Autodesk Inventor part; units mm, degrees
ref_plane "YZ Plane" through (0, 0, 0) normal (1, 0, 0) x (0, 1, 0)
ref_plane "XZ Plane" through (0, 0, 0) normal (0, 1, 0) x (-1, 0, 0)
ref_plane "XY Plane" through (0, 0, 0) normal (0, 0, 1) x (1, 0, 0)
sketch "Sketch3" plane through (0, 0, 0) normal (0, 1, 0) x (-1, 0, 0)
  line L0 (0.305195, 0) -> (-44.144805, 0)
  line L1 (-44.144805, 0) -> (-44.144805, -19.05)
  line L2 (-44.144805, -19.05) -> (0.305195, -19.05)
  line L3 (0.305195, -19.05) -> (0.305195, 0)
  arc A0 (-5.25, -6.73951) -> (-5.25, -5.26049) centre (-3.125, -6) ccw
  circle A1 centre (-3.125, -6) radius 2.25
  arc A2 (35.25, -5.26049) -> (35.25, -6.73951) centre (33.125, -6) ccw
  circle A3 centre (33.125, -6) radius 2.25
  line L4 (33.125, -6) -> (-3.125, -6)
  line L5 (0, -12) -> (0, 0)
  line L6 (30, -12) -> (0, -12)
  line L7 (0, -12) -> (0, 0)
  line L8 (0, 0) -> (30, 0)
  line L9 (30, 0) -> (30, -12)
  line L10 (30, -12) -> (0, 0) construction
  line L11 (0, -12) -> (30, 0) construction
  arc A4 (-42.475, -10.26451) -> (-42.475, -8.78549) centre (-40.35, -9.525) ccw
  circle A5 centre (-40.35, -9.525) radius 2.25
  arc A6 (-1.975, -8.78549) -> (-1.975, -10.26451) centre (-4.1, -9.525) ccw
  circle A7 centre (-4.1, -9.525) radius 2.25
  line L12 (-4.1, -9.525) -> (-40.35, -9.525)
  line L13 (-37.225, -15.525) -> (-37.225, -3.525)
  line L14 (-7.225, -15.525) -> (-37.225, -15.525)
  line L15 (-37.225, -15.525) -> (-37.225, -3.525)
  line L16 (-37.225, -3.525) -> (-7.225, -3.525)
  line L17 (-7.225, -3.525) -> (-7.225, -15.525)
  line L18 (-7.225, -15.525) -> (-37.225, -3.525) construction
  line L19 (-37.225, -15.525) -> (-7.225, -3.525) construction
  point P0 (15, -6)
  point P1 (-22.225, -9.525)
  point P2 (-4.875952, -7.413035)
  point P3 (-5.25, -6.73951)
  point P4 (-2.349048, -8.111965)
  point P5 (-1.975, -10.26451)
  point P6 (0.305195, -12)
  dimension "d12" = 4.5
  dimension "d13" = 4.5
  dimension "d17" = 4.5
  dimension "d18" = 4.5
  dimension "d9" = 44.45
  dimension "d10" = 19.05
  dimension "d11" = 36.25
  dimension "d14" = 30
  dimension "d15" = 12
  dimension "d16" = 36.25
  dimension "d19" = 30
  dimension "d20" = 12
extrude "Extrusion2" add sketch "Sketch3" along normal blind 3.81 contours L5 L6 L3 L2 L1 L0 | A0 A6 A1
sketch "Sketch4" plane through (0, 3.81, 0) normal (0, 1, 0) x (1, 0, 0)
  line L0 (0, 12) -> (0, 0)
  line L1 (-0.305195, 19.05) -> (-0.305195, 12)
  line L2 (0, 12) -> (-0.305195, 12)
  line L3 (-0.305195, 12) -> (-0.305195, 19.05)
  line L4 (-0.305195, 19.05) -> (0, 19.05)
  line L5 (0, 19.05) -> (0, 12)
extrude "Extrusion3" cut sketch "Sketch4" against normal blind 3.81
sketch "Sketch5" plane through (0, 3.81, 0) normal (0, 1, 0) x (1, 0, 0)
  line L0 (44.144805, 19.05) -> (0, 19.05)
  line L1 (22.072403, 19.05) -> (22.072403, 0)
  line L2 (0, 0) -> (44.144805, 0)
  line L3 (22.072403, 9.525) -> (0, 9.525)
  line L4 (0, 19.05) -> (0, 0)
  circle A0 centre (3.999998, -4) radius 4
  circle A1 centre (3.999998, -4) radius 1.5
  line L5 (0, 0) -> (44.144805, 0)
  line L6 (0, -4.004242) -> (0, 0)
  line L7 (0, 0) -> (7.846401, 0)
  line L8 (7.846401, 0) -> (7.999998, -4.001295)
  circle A2 centre (3.999998, 23.05) radius 4
  circle A3 centre (3.999998, 23.05) radius 1.5
  line L9 (0, 23.054242) -> (0, 19.05)
  line L10 (0, 19.05) -> (7.846401, 19.05)
  line L11 (7.846401, 19.05) -> (7.999998, 23.051295)
  line L12 (44.144805, 19.05) -> (44.144805, 0)
  circle A4 centre (40.144808, -4) radius 4
  circle A5 centre (40.144808, -4) radius 1.5
  line L13 (44.144805, -4.004242) -> (44.144805, 0)
  line L14 (44.144805, 0) -> (36.298405, 0)
  line L15 (36.298405, 0) -> (36.144808, -4.001295)
  circle A6 centre (40.144808, 23.05) radius 4
  circle A7 centre (40.144808, 23.05) radius 1.5
  line L16 (44.144805, 23.054242) -> (44.144805, 19.05)
  line L17 (44.144805, 19.05) -> (36.298405, 19.05)
  line L18 (36.298405, 19.05) -> (36.144808, 23.051295)
  point P0 (44.144805, 9.525)
  point P1 (7.846401, 0)
  dimension "d25" = 8
  dimension "d26" = 3
sketch "Sketch5 outline for Extrusion4" plane through (0, 3.81, 0) normal (0, 1, 0) x (1, 0, 0)
  line L0 (44.144805, -4.004242) -> (44.144805, 0)
  arc A0 (36.144808, -4.001295) -> (44.144805, -4.004242) centre (40.144808, -4) ccw
  line L1 (44.144805, 0) -> (36.298405, 0)
  line L2 (36.298405, 0) -> (36.144808, -4.001295)
  circle A1 centre (40.144808, -4) radius 1.5
  line L3 (36.298405, 19.05) -> (44.144805, 19.05)
  line L4 (36.144808, 23.051295) -> (36.298405, 19.05)
  line L5 (44.144805, 19.05) -> (44.144805, 23.054242)
  arc A2 (44.144805, 23.054242) -> (36.144808, 23.051295) centre (40.144808, 23.05) ccw
  circle A3 centre (40.144808, 23.05) radius 1.5
  line L6 (0, 0) -> (0, -4.004242)
  line L7 (7.846401, 0) -> (0, 0)
  arc A4 (0, -4.004242) -> (7.999998, -4.001295) centre (3.999998, -4) ccw
  line L8 (7.999998, -4.001295) -> (7.846401, 0)
  circle A5 centre (3.999998, -4) radius 1.5
  line L9 (7.846401, 19.05) -> (7.999998, 23.051295)
  line L10 (0, 19.05) -> (7.846401, 19.05)
  arc A6 (7.999998, 23.051295) -> (0, 23.054242) centre (3.999998, 23.05) ccw
  line L11 (0, 23.054242) -> (0, 19.05)
  circle A7 centre (3.999998, 23.05) radius 1.5
extrude "Extrusion4" add sketch "Sketch5 outline for Extrusion4" against normal blind 3.81
sketch "Sketch6" plane through (0, 3.81, 0) normal (0, 1, 0) x (1, 0, 0)
  line L0 (0, -7.9375) -> (44.144805, -7.9375)
  line L1 (44.144805, -7.9375) -> (44.144805, 26.9875)
  line L2 (44.144805, 26.9875) -> (0, 26.9875)
  line L3 (0, 26.9875) -> (0, -7.9375)
  circle A0 centre (3.999998, 23.05) radius 1.5
  circle A1 centre (3.999998, 23.05) radius 1.5
  circle A2 centre (3.999998, -4) radius 1.5
  circle A3 centre (3.999998, -4) radius 1.5
  circle A4 centre (40.144808, -4) radius 1.5
  circle A5 centre (40.144808, -4) radius 1.5
  circle A6 centre (40.144808, 23.05) radius 1.5
  circle A7 centre (40.144808, 23.05) radius 1.5
properties part number "motor mount v2"
Design review of the part built by this model. Coordinates are the model's own, in mm. A direction names the side the tool comes from. Give positions to 0.01 mm unless a question says otherwise; leave off trailing zeros. Write each loop counter-clockwise with the first axis right and the second up, starting at its lowest first coordinate (ties: lowest second). Pieces come first, ordered by that corner, then holes. Notation, with made-up numbers: M 11,7 L 54,7 A19 ccw 54,21 Z; hole C -14.5,10.25 d3. An arc over 180 degrees is marked long. Answer as a JSON object with one key per item and string values. Group by question number.
1) For line 1 along X through (y, z) = (2.05, 4); line 2 along Z through (x, y) = (35.5, 1.55) (3 decimals); line 3 along X through (y, z) = (1.65, -22.5), list the stretches that pass through material, from the lowest coordinate up.
2) We need section A-A (z = -13). Give the boundary of the cut face in (x, y) (3 decimals).
3) Clearance check with flat-ended pins moving along their axes: pin 1 Ø2.5 at (x, z) = (40.14, -23.05) entering from -Y; pin 2 Ø1.1 at (x, y) = (17, 1.5) entering from +Z; pin 3 Ø1.9 at (x, y) = (28.5, 3) entering from -Z. State where each tip first meets the part, or that it passes through.
4) We need section C-C (x = 40.35). Give the boundary of the cut face in (y, z) (3 decimals), and give its area (3 significant figures).
5) Mouldability with a two-part tool opening along X and no side actions: class faces 3 (the face through (22, 3.81, -17)), 4 (the face through (36.223, 1.932, 1.973)), 5 (the face through (44.145, 2, -9)) as released by +X, released by -X, zero draft, split by the parting line, or undercut.
6) We need section D-D (y = 2.4). Count the separate pieces of the cut face and the enclosed holes in it, and give its area (3 significant figures).
7) Tool access review of faces 1 (the face through (22, 0, -17)), 2 (the face through (7.924, 1.932, 2.029)): name each direction out of +Z, -Z, +X, -X, +Y, -Y from which nothing blocks a thin tool from reaching the whole face with its end or side.
8) We need section B-B (x = 23.5). Give the boundary of the cut face in (y, z) (3 decimals).
Answer key:
{
 "1": {"line 1": "x = 0 to 2.5, 5.5 to 8, 36.14 to 38.64, 41.64 to 44.14", "line 2": "z = -19.05 to -15.525, -3.525 to 0", "line 3": "x = 0 to 2.6, 5.4 to 7.98, 36.17 to 38.75, 41.54 to 44.14"},
 "2": {"outline": "M 0,0 L 7.225,0 L 7.225,3.81 L 0,3.81 Z; M 37.225,0 L 44.145,0 L 44.145,3.81 L 37.225,3.81 Z"},
 "3": {"pin 1": "passes through", "pin 2": "stops at z = 0", "pin 3": "stops at z = -19.05"},
 "4": {"outline": "M 0,-27.045 L 3.81,-27.045 L 3.81,-24.536 L 0,-24.536 Z; M 0,-21.564 L 3.81,-21.564 L 3.81,-11.775 L 0,-11.775 Z; M 0,-7.275 L 3.81,-7.275 L 3.81,2.514 L 0,2.514 Z; M 0,5.486 L 3.81,5.486 L 3.81,7.995 L 0,7.995 Z", "area": "93.7 mm²"},
 "5": {"face 3": "zero draft", "face 4": "undercut", "face 5": "released by +X"},
 "6": {"separate pieces": "1", "enclosed holes": "7", "area": "648 mm²"},
 "7": {"face 1": "+Z, -Z, +X, -X, -Y", "face 2": "+Y, -Y"},
 "8": {"outline": "M 0,-19.05 L 3.81,-19.05 L 3.81,-15.525 L 0,-15.525 Z; M 0,-3.525 L 3.81,-3.525 L 3.81,0 L 0,0 Z"}
}
